The model under review builds one solid part; all positions refer to its coordinate system, in mm. A direction names the side the tool comes from. Coordinates: 2 decimals unless noted, no trailing zeros. Order: outer loops, then holes, each group sorted by start corner. A loop starts at its lowest first (then second) coordinate and runs counter-clockwise, first axis right, second up. Notation, with made-up numbers: M 16,-29 L 75,-29 A19 cw 75,2 Z; hole C 18.5,76 d10. An arc over 180 degrees is marked long. Answer in a Markdown table with one row per item.
from build123d import *

# Parameters (mm, degrees)
ESQUISSE1_W             = 128
ESQUISSE1_H             = 53
ESQUISSE1_W_2           = 122
ESQUISSE1_H_2           = 47
BOSS_EXTRU_1_DEPTH      = 25
ESQUISSE2_W             = 128
ESQUISSE2_H             = 53
BOSS_EXTRU_2_DEPTH      = 3
BOSS_EXTRU_3_DEPTH      = 25
ENL_V_MAT_EXTRU_1_DEPTH = 3
ESQUISSE5_R             = 1
ENL_V_MAT_EXTRU_2_DEPTH = 20
CONG_1_R                = 5
CONG_2_R                = 5
ESQUISSE6_W             = 28
ESQUISSE6_H             = 5
ENL_V_MAT_EXTRU_3_DEPTH = 3
ENL_V_MAT_EXTRU_4_DEPTH = 8
ENL_V_MAT_EXTRU_6_DEPTH = 8
ENL_V_MAT_EXTRU_7_DEPTH = 8
ESQUISSE13_W            = 2
ESQUISSE13_H            = 6
ENL_V_MAT_EXTRU_8_DEPTH = 3
CONG_4_R                = 2
CONG_5_R                = 2


with BuildPart() as part:
    # Esquisse1 → Boss.-Extru.1 (new body)
    with BuildSketch(Plane.XY):
        Rectangle(ESQUISSE1_W, ESQUISSE1_H)
        Rectangle(ESQUISSE1_W_2, ESQUISSE1_H_2, mode=Mode.SUBTRACT)
    extrude(amount=BOSS_EXTRU_1_DEPTH)

    # Esquisse2 → Boss.-Extru.2 (add)
    with BuildSketch(Plane.XY.offset(25)):
        Rectangle(ESQUISSE2_W, ESQUISSE2_H)
    extrude(amount=BOSS_EXTRU_2_DEPTH)

    # Esquisse3 → Boss.-Extru.3 (add)
    with BuildSketch(Plane(origin=(0, 0, 25), x_dir=(-1, 0, 0), z_dir=(0, 0, -1))):
        Polygon((61, 23.5), (56, 23.5), (61, 18.5), align=None)
        Polygon((61, -23.5), (61, -18.5), (56, -23.5), align=None)
        Polygon((-61, -23.5), (-61, -18.5), (-56, -23.5), align=None)
        Polygon((-61, 18.5), (-56, 23.5), (-61, 23.5), align=None)
    extrude(amount=BOSS_EXTRU_3_DEPTH)

    # Esquisse4 → Enlèv. mat.-Extru.1 (cut)
    with BuildSketch(Plane.XY.offset(28)):
        with BuildLine():
            Line((-44, 18.5), (-44, -16.5))
            ThreePointArc((-44, -16.5), (-42.5, -18), (-41, -16.5))
            Line((-41, -16.5), (-41, 18.5))
            ThreePointArc((-41, 18.5), (-42.5, 20), (-44, 18.5))
        make_face()
        with BuildLine():
            Line((-23, 18.5), (-23, -16.5))
            ThreePointArc((-23, -16.5), (-21.5, -18), (-20, -16.5))
            Line((-20, -16.5), (-20, 18.5))
            ThreePointArc((-20, 18.5), (-21.5, 20), (-23, 18.5))
        make_face()
        with BuildLine():
            Line((-2, 18.5), (-2, -16.5))
            ThreePointArc((-2, -16.5), (-0.5, -18), (1, -16.5))
            Line((1, -16.5), (1, 18.5))
            ThreePointArc((1, 18.5), (-0.5, 20), (-2, 18.5))
        make_face()
        with BuildLine():
            Line((19, 18.5), (19, -16.5))
            ThreePointArc((19, -16.5), (20.5, -18), (22, -16.5))
            Line((22, -16.5), (22, 18.5))
            ThreePointArc((22, 18.5), (20.5, 20), (19, 18.5))
        make_face()
        with BuildLine():
            Line((40, 18.5), (40, -16.5))
            ThreePointArc((40, -16.5), (41.5, -18), (43, -16.5))
            Line((43, -16.5), (43, 18.5))
            ThreePointArc((43, 18.5), (41.5, 20), (40, 18.5))
        make_face()
    extrude(amount=-ENL_V_MAT_EXTRU_1_DEPTH, mode=Mode.SUBTRACT)

    # Esquisse5 → Enlèv. mat.-Extru.2 (cut)
    with BuildSketch(Plane(origin=(0, 0, 0), x_dir=(-1, 0, 0), z_dir=(0, 0, -1))):
        with Locations((-60.621320344, 23.121320344)):
            Circle(ESQUISSE5_R)
        with Locations((60.621320344, 23.121320344)):
            Circle(ESQUISSE5_R)
        with Locations((-60.621320344, -23.121320344)):
            Circle(ESQUISSE5_R)
        with Locations((60.621320344, -23.121320344)):
            Circle(ESQUISSE5_R)
    extrude(amount=-ENL_V_MAT_EXTRU_2_DEPTH, mode=Mode.SUBTRACT)

    # Congé1
    cong_1_edges = [part.edges().sort_by_distance(p)[0] for p in [
        (56, 23.5, 12.5),
    ]]
    fillet(cong_1_edges, radius=CONG_1_R)

    # Congé2
    cong_2_edges = [part.edges().sort_by_distance(p)[0] for p in [
        (-56, 23.5, 12.5),
        (-61, 18.5, 12.5),
        (-56, -23.5, 12.5),
        (-61, -18.5, 12.5),
        (56, -23.5, 12.5),
        (61, -18.5, 12.5),
        (61, 18.5, 12.5),
    ]]
    fillet(cong_2_edges, radius=CONG_2_R)

    # Esquisse6 → Enlèv. mat.-Extru.3 (cut)
    with BuildSketch(Plane(origin=(64, 0, 0), x_dir=(0, 0, -1), z_dir=(1, 0, 0))):
        with Locations((-14, 14)):
            Rectangle(ESQUISSE6_W, ESQUISSE6_H)
    extrude(amount=-ENL_V_MAT_EXTRU_3_DEPTH, mode=Mode.SUBTRACT)

    # Esquisse7 → Enlèv. mat.-Extru.4 (cut)
    with BuildSketch(Plane(origin=(0, 26.5, 0), x_dir=(1, 0, 0), z_dir=(0, 1, 0))):
        with BuildLine():
            Line((-9, 0), (-4, 0))
            Line((-4, 0), (-4, -5))
            ThreePointArc((-4, -5), (-6.5, -7.5), (-9, -5))
            Line((-9, -5), (-9, 0))
        make_face()
    extrude(amount=-ENL_V_MAT_EXTRU_4_DEPTH, mode=Mode.SUBTRACT)

    # Esquisse9 → Enlèv. mat.-Extru.6 (cut)
    with BuildSketch(Plane.XZ.offset(26.5)):
        with BuildLine():
            Line((44, 0), (49, 0))
            Line((49, 0), (49, 5))
            ThreePointArc((49, 5), (46.5, 7.5), (44, 5))
            Line((44, 5), (44, 0))
        make_face()
    extrude(amount=-ENL_V_MAT_EXTRU_6_DEPTH, mode=Mode.SUBTRACT)

    # Esquisse10 → Enlèv. mat.-Extru.7 (cut)
    with BuildSketch(Plane.XY.offset(28)):
        with BuildLine():
            Line((61, 16.5), (60, 16.5))
            ThreePointArc((60, 16.5), (57.5, 14), (60, 11.5))
            Line((60, 11.5), (61, 11.5))
            Line((61, 11.5), (61, 16.5))
        make_face()
    extrude(amount=-ENL_V_MAT_EXTRU_7_DEPTH, mode=Mode.SUBTRACT)

    # Esquisse13 → Enlèv. mat.-Extru.8 (cut)
    with BuildSketch(Plane.ZY.offset(64)):
        with Locations((1, 0)):
            Rectangle(ESQUISSE13_W, ESQUISSE13_H)
    extrude(amount=-ENL_V_MAT_EXTRU_8_DEPTH, mode=Mode.SUBTRACT)

    # Congé4
    cong_4_edges = [part.edges().sort_by_distance(p)[0] for p in [
        (60.60568242, 18.375130905, 25),
        (58.5, 21, 25),
        (55.84234935, 23.119397663, 25),
        (61, -2.464466094, 25),
        (60.619397663, -18.34234935, 25),
        (58.5, -21, 25),
        (55.84234935, -23.119397663, 25),
        (0, -23.5, 25),
        (-55.84234935, -23.119397663, 25),
        (-58.5, -21, 25),
        (-60.619397663, -18.34234935, 25),
        (-61, 0, 25),
        (-60.619397663, 18.34234935, 25),
        (-58.5, 21, 25),
        (-55.84234935, 23.119397663, 25),
        (0, 23.5, 25),
    ]]
    fillet(cong_4_edges, radius=CONG_4_R)

    # Congé5
    cong_5_edges = [part.edges().sort_by_distance(p)[0] for p in [
        (-64, 26.5, 14),
        (64, 26.5, 14),
        (64, -26.5, 14),
        (-64, -26.5, 14),
    ]]
    fillet(cong_5_edges, radius=CONG_5_R)


solid = part.part
(1) To check wall thickness, follow line 1 (X direction, y = 6.5, z = 9); line 2 (Y direction, x = -21, z = 9.5); line 3 (X direction, y = 9, z = 26.75). State the ranges of each line that lie inside material, in increasing order. Write a range as [from, to].
Report:
| item | result |
|---|---|
| line 1 | [-64, -61], [61, 64] |
| line 2 | [-26.5, -23.5], [23.5, 26.5] |
| line 3 | [-64, -44], [-41, -23], [-20, -2], [1, 19], [22, 40], [43, 64] |
(2) Machinability: for faces 4 (the flat face through (64, -7, 14)), 5 (the flat face through (40, 1, 27)), 6 (the flat face through (-61, 0, 11)), which of the approach directions +Z, -Z, +X, -X, +Y, -Y give a long, thin tool a straight path to every point of the face, cutting with its end or side? Answer none if there is none.
Report:
| item | result |
|---|---|
| face 4 | +Z, -Z, +X, +Y, -Y |
| face 5 | +Z, -Z |
| face 6 | -Z |
(3) Insertion check: P1, Ø1, axis at x = -60.5, y = 23, coming from the -Z side. The pin has a flat end and moves straight along its axis. Give the tip position at first contact, or say it passes through.
Report:
| item | result |
|---|---|
| P1 | z = 20 |
(4) Take a section at B-B (x = -0.5). Write out the cut boundary in (y, z).
Report:
| item | result |
|---|---|
| outline | M -26.5,0 L -23.5,0 L -23.5,23 A2 cw -21.5,25 L -18,25 L -18,28 L -26.5,28 Z; M 20,25 L 21.5,25 A2 cw 23.5,23 L 23.5,0 L 26.5,0 L 26.5,28 L 20,28 Z |
(5) The part is to be moulded in two halves that separate along Y. For faces 1 (the cylindrical face through (-42.5, -18, 26.5)), 2 (the flat face through (49, -25, 2)), 3 (the flat face through (-1, -26.5, 14)), say which applies: +Y half, -Y half, draft (parallel to the pull), parting line (faces both ways), or undercut.
Report:
| item | result |
|---|---|
| face 1 | undercut |
| face 2 | draft |
| face 3 | -Y half |
(6) Take a section at D-D (y = 14). Write out the cut boundary in (x, z).
Report:
| item | result |
|---|---|
| outline | M -64,0 L -61,0 L -61,23 A2 cw -59,25 L -44,25 L -44,28 L -64,28 Z; M -41,25 L -23,25 L -23,28 L -41,28 Z; M -20,25 L -2,25 L -2,28 L -20,28 Z; M 1,25 L 19,25 L 19,28 L 1,28 Z; M 22,25 L 40,25 L 40,28 L 22,28 Z; M 43,25 L 57.5,25 L 57.5,28 L 43,28 Z |
(7) Take a section at A-A (y = -10). State how many separate pieces and enclosed holes the cut face has, then the cut area to 3 significant figures.
Report:
| item | result |
|---|---|
| separate pieces | 6 |
| enclosed holes | 0 |
| area | 491 mm^2 |
(8) Take a section at C-C (z = 21.5). Write out the cut boundary in (x, y), then the cut area to 3 significant figures.
Report:
| item | result |
|---|---|
| outline | M -64,-24.5 A2 ccw -62,-26.5 L 62,-26.5 A2 ccw 64,-24.5 L 64,11.5 L 61,11.5 L 61,-16.43 A5 cw 59.54,-19.96 L 57.46,-22.04 A5 cw 53.93,-23.5 L -53.93,-23.5 A5 cw -57.46,-22.04 L -59.54,-19.96 A5 cw -61,-16.43 L -61,16.43 A5 cw -59.54,19.96 L -57.46,22.04 A5 cw -53.93,23.5 L 53.93,23.5 A5 cw 57.46,22.04 L 59.54,19.96 A5 cw 61,16.5 L 64,16.5 L 64,24.5 A2 ccw 62,26.5 L -62,26.5 A2 ccw -64,24.5 Z |
| area | 1,090 mm^2 |
